Part model, mm, in its own coordinate system. Face numbers are marked on the shaded views. Round coordinates to 2 decimals unless told otherwise and drop trailing zeros. Write each loop counter-clockwise with the first axis right and the second up, starting at its lowest first coordinate (ties: lowest second). Pieces come first, ordered by that corner, then holes. Notation, with made-up numbers: (21, 59.5) -> (68, 59.5) arc R24 ccw to (68, 92.5) -> close; hole circle Ø4 at (-2.5, 2). An arc over 180 degrees is marked (long way). Return JSON: item names as keys, results as strings. Group by question number.
Autodesk Inventor part; units mm, degrees
ref_plane "YZ Plane" through (0, 0, 0) normal (1, 0, 0) x (0, 1, 0)
ref_plane "XZ Plane" through (0, 0, 0) normal (0, 1, 0) x (-1, 0, 0)
ref_plane "XY Plane" through (0, 0, 0) normal (0, 0, 1) x (1, 0, 0)
sketch "스케치1" plane through (0, 0, 0) normal (0, 0, 1) x (1, 0, 0)
  line L0 (0, 0) -> (10, 0)
  line L1 (10, 0) -> (10, 12.5)
  line L2 (10, 12.5) -> (0, 12.5)
  line L3 (0, 12.5) -> (0, 0)
  line L4 (-1.5, 14) -> (11.5, 14)
  line L5 (11.5, 14) -> (11.5, -1.5)
  line L6 (11.5, -1.5) -> (-1.5, -1.5)
  line L7 (-1.5, -1.5) -> (-1.5, 14)
  line L8 (0, 0) -> (0, -1.5)
  line L9 (10, 0) -> (10, -1.5)
  line L10 (0, 0) -> (-1.5, 0)
  line L11 (10, 0) -> (11.5, 0)
  dimension "d0" = 10
  dimension "d1" = 12.5
  dimension "d2" = 1.5
extrude "돌출1" add sketch "스케치1" along normal blind 20 contours L10 L7 L4 L5 L11 L1 L2 L3 | L8 L6 L7 L10 | L11 L5 L6 L9
sketch "스케치2" plane through (-1.5, -1.5, 0) normal (0, -1, 0) x (1, 0, 0)
  line L0 (0, 0) -> (1.5, 0)
  line L1 (1.5, 0) -> (1.5, 20)
  line L2 (0, 20) -> (1.5, 20)
  line L3 (0, 0) -> (0, 20)
  line L4 (1.5, 5.5) -> (0, 5.5)
  line L5 (0, 5.5) -> (0, 6)
  line L6 (0, 6) -> (1.5, 6)
  line L7 (1.5, 6) -> (1.5, 5.5)
  point P0 (1.5, 0)
  point P1 (1.5, 6)
  point P2 (0, 5.5)
  dimension "d5" = 0.5
  dimension "d6" = 5.5
extrude "돌출2" cut sketch "스케치2" against normal blind 8 contours L3 L6 L1 L4
fillet "모깎기1" radius 2 2 edges at (-1.5, 14, 10) (11.5, 14, 10)
sketch "스케치3" plane through (10, -1.5, 0) normal (0, -1, 0) x (1, 0, 0)
  line L0 (-10.75, 19) -> (0.75, 19)
  line L1 (0.75, 19) -> (0.75, 18)
  line L2 (0.75, 18) -> (-10.75, 18)
  line L3 (-10.75, 18) -> (-10.75, 19)
  line L4 (-11.5, 6) -> (-10, 6)
  line L5 (-10, 6) -> (-10, 20)
  line L6 (-11.5, 20) -> (-10, 20)
  line L7 (-11.5, 6) -> (-11.5, 20)
  line L8 (0, 0) -> (1.5, 0)
  line L9 (1.5, 0) -> (1.5, 20)
  line L10 (0, 20) -> (1.5, 20)
  line L11 (0, 0) -> (0, 20)
  point P0 (-10, 0)
  point P1 (-10.75, 20)
  point P2 (-10.75, 18.5)
  point P3 (0.75, 20)
  point P4 (0.75, 18.5)
  dimension "d10" = 1
  dimension "d11" = 1
extrude "돌출3" cut sketch "스케치3" against normal blind 14.5 contours L0 L5 L2 L3 | L0 L11 L2 L5 | L0 L1 L2 L11
sketch "스케치4" plane through (0, -1.5, 0) normal (1, 0, 0) x (0, 0, -1)
  line L0 (-2.8, 5.5) -> (-1.8, 5.5)
  line L1 (-1.8, 5.5) -> (-1.8, 8.5)
  line L2 (-1.8, 8.5) -> (-2.8, 8.5)
  line L3 (-2.8, 8.5) -> (-2.8, 5.5)
  line L4 (0, 0) -> (-5.5, 0)
  line L5 (0, 13.5) -> (0, 0)
  point P0 (0, 1.5)
  point P1 (-2.8, 7)
  dimension "d14" = 1
  dimension "d15" = 3
  dimension "d16" = 7
  dimension "d20" = 2.8
extrude "돌출4" add sketch "스케치4" along normal blind 2
properties part number "_3D 인쇄"
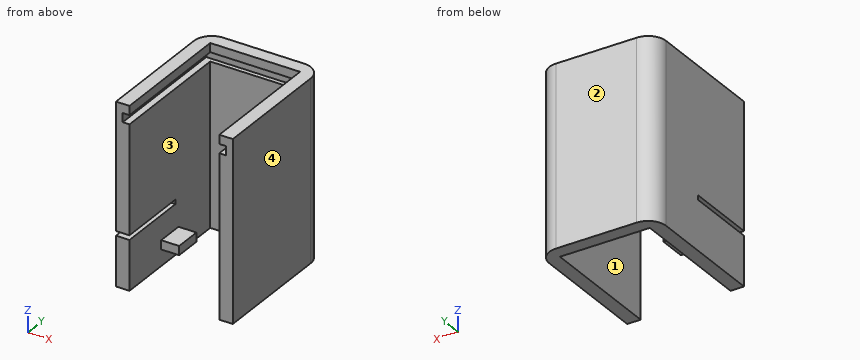
Item 1: Cut at A-A (y = 1). Write the cut outline in (x, z).
Item 2: Cut at B-B (x = 1.25). Write the cut outline in (y, z).
Item 3: Cut at D-D (x = 6). Write the cut outline in (y, z).
Item 4: Two-plate mould, pull along X, no slides. Class the marked faces 1, 2, 3 and 4: released by +X, released by -X, zero draft, split by the parting line, or undercut.
Item 5: Cut at C-C (y = 11.5). Write the cut outline in (x, z).
Item 6: Flat gauge pins, fed straight in: P1, Ø3, axis at x = 8, z = 10.5, coming from the -Y side; P2, Ø1.6, axis at x = 1, y = 5.5, coming from the -Z side. Where does each tip first touch, or does it go through?
Item 7: Wall check: L1, parallel to X at y = 9.75, z = 15.25; L2, parallel to Y at x = 7, z = 14; L3, parallel to X at y = 12.75, z = 10. Give the ranges that are in metal, low to high.
Checks:
{
 "1": {"outline": "(-1.5, 0) -> (0, 0) -> (0, 5.5) -> (-1.5, 5.5) -> close; (-1.5, 6) -> (0, 6) -> (0, 18) -> (-0.75, 18) -> (-0.75, 19) -> (0, 19) -> (0, 20) -> (-1.5, 20) -> close; (10, 0) -> (11.5, 0) -> (11.5, 20) -> (10, 20) -> (10, 19) -> (10.75, 19) -> (10.75, 18) -> (10, 18) -> close"},
 "2": {"outline": "(4, 1.8) -> (7, 1.8) -> (7, 2.8) -> (4, 2.8) -> close; (12.5, 0) -> (14, 0) -> (14, 20) -> (12.5, 20) -> (12.5, 19) -> (13, 19) -> (13, 18) -> (12.5, 18) -> close"},
 "3": {"outline": "(12.5, 0) -> (14, 0) -> (14, 20) -> (12.5, 20) -> (12.5, 19) -> (13, 19) -> (13, 18) -> (12.5, 18) -> close"},
 "4": {"face 1": "undercut", "face 2": "zero draft", "face 3": "undercut", "face 4": "released by +X"},
 "5": {"outline": "(-1.5, 0) -> (0, 0) -> (0, 18) -> (-0.75, 18) -> (-0.75, 19) -> (0, 19) -> (0, 20) -> (-1.5, 20) -> close; (10, 0) -> (11.5, 0) -> (11.5, 20) -> (10, 20) -> (10, 19) -> (10.75, 19) -> (10.75, 18) -> (10, 18) -> close"},
 "6": {"P1": "stops at y = 12.5", "P2": "stops at z = 1.8"},
 "7": {"L1": "x = -1.5 to 0, 10 to 11.5", "L2": "y = 12.5 to 14", "L3": "x = -1.35 to 11.35"}
}
